```python
from build123d import *

# Parameters (mm, degrees)
SKETCH1_R           = 35
BOSS_EXTRUDE1_DEPTH = 150
FILLET1_R           = 1
CUT_EXTRUDE1_START  = -10
SKETCH3_R           = 35
SKETCH3_R_2         = 34
CUT_EXTRUDE1_DEPTH  = 10
BOSS_EXTRUDE2_START = -5
SKETCH4_R           = 2.25
BOSS_EXTRUDE2_DEPTH = 6
BOSS_EXTRUDE3_DEPTH = 64


with BuildPart() as part:
    # Sketch1 → Boss-Extrude1 (new body)
    with BuildSketch(Plane(origin=(0, 0, 0), x_dir=(1, 0, 0), z_dir=(0, 1, 0))):
        with Locations(Location((0, 0, 0), (0, 0, 270))):
            Circle(SKETCH1_R)
        with BuildLine():
            Line((-31.448370387, -10), (31.448370387, -10))
            ThreePointArc((31.448370387, -10), (0, 33), (-31.448370387, -10))
        make_face(mode=Mode.SUBTRACT)
        with BuildLine():
            Line((-30.740852298, -12), (30.740852298, -12))
            ThreePointArc((30.740852298, -12), (0, -33), (-30.740852298, -12))
        make_face(mode=Mode.SUBTRACT)
    extrude(amount=BOSS_EXTRUDE1_DEPTH)

    # Fillet1
    fillet1_edges = [part.edges().sort_by_distance(p)[0] for p in [
        (-30.740852298, 75, 12),
        (30.740852298, 75, 12),
        (31.448370387, 75, 10),
        (-31.448370387, 75, 10),
    ]]
    fillet(fillet1_edges, radius=FILLET1_R)

    # Sketch3 → Cut-Extrude1 (cut)
    # profile 1 of 2: a face of its own
    with BuildSketch(Plane(origin=(0, 150, 0), x_dir=(1, 0, 0), z_dir=(0, 1, 0)).offset(CUT_EXTRUDE1_START)):
        with Locations(Location((0, 0, 0), (0, 0, 270))):
            Circle(SKETCH3_R)
        with Locations(Location((0, 0, 0), (0, 0, 270))):
            Circle(SKETCH3_R_2, mode=Mode.SUBTRACT)
    # profile 2 of 2: a face of its own
    with BuildSketch(Plane(origin=(0, 150, 0), x_dir=(1, 0, 0), z_dir=(0, 1, 0)).offset(CUT_EXTRUDE1_START)):
        with BuildLine():
            Line((30.708305066, -10), (-30.708305066, -10))
            ThreePointArc((-30.708305066, -10), (-31.307784006, -9.80039053), (-31.667939599, -9.28125))
            ThreePointArc((-31.667939599, -9.28125), (-31.402080367, -10.144424508), (-31.112698372, -11))
            Line((-31.112698372, -11), (31.112698372, -11))
            ThreePointArc((31.112698372, -11), (31.402080367, -10.144424508), (31.667939599, -9.28125))
            ThreePointArc((31.667939599, -9.28125), (31.307784006, -9.80039053), (30.708305066, -10))
        make_face()
    extrude(amount=CUT_EXTRUDE1_DEPTH, mode=Mode.SUBTRACT)

    # Sketch4 → Boss-Extrude2 (add)
    with BuildSketch(Plane.XZ.offset(BOSS_EXTRUDE2_START)):
        with BuildLine():
            Line((-23.25, 10), (23.25, 10))
            Line((23.25, 10), (23.25, 0))
            ThreePointArc((23.25, 0), (19.66205807, -8.66205807), (11, -12.25))
            Line((11, -12.25), (7.5, -10.75))
            Line((7.5, -10.75), (-7.5, -10.75))
            Line((-7.5, -10.75), (-11, -12.25))
            ThreePointArc((-11, -12.25), (-19.66205807, -8.66205807), (-23.25, 0))
            Line((-23.25, 0), (-23.25, 10))
        make_face()
        with Locations(Location((0, -7.5, 0), (0, 0, 270))):
            Circle(SKETCH4_R, mode=Mode.SUBTRACT)
        with Locations(Location((20.5, 7.5, 0), (0, 0, 270))):
            Circle(SKETCH4_R, mode=Mode.SUBTRACT)
        with Locations(Location((-20.5, 7.5, 0), (0, 0, 270))):
            Circle(SKETCH4_R, mode=Mode.SUBTRACT)
        with Locations(Location((0, 7.5, 0), (0, 0, 270))):
            Circle(SKETCH4_R, mode=Mode.SUBTRACT)
        with BuildLine():
            Line((-3, 4.643543905), (3, 4.643543905))
            ThreePointArc((3, 4.643543905), (20.25, 0), (3, -4.643543905))
            Line((3, -4.643543905), (-3, -4.643543905))
            ThreePointArc((-3, -4.643543905), (-20.25, 0), (-3, 4.643543905))
        make_face(mode=Mode.SUBTRACT)
    extrude(amount=-BOSS_EXTRUDE2_DEPTH)

    # Sketch5 → Boss-Extrude3 (add)
    with BuildSketch(Plane(origin=(0, 11, 0), x_dir=(1, 0, 0), z_dir=(0, 1, 0))):
        with BuildLine():
            Line((-23.25, 0), (-23.25, -10))
            Line((-23.25, -10), (23.25, -10))
            Line((23.25, -10), (23.25, 0))
            ThreePointArc((23.25, 0), (19.66205807, 8.66205807), (11, 12.25))
            Line((11, 12.25), (7.5, 10.75))
            Line((7.5, 10.75), (-7.5, 10.75))
            Line((-7.5, 10.75), (-11, 12.25))
            ThreePointArc((-11, 12.25), (-19.66205807, 8.66205807), (-23.25, 0))
        make_face()
        with BuildLine():
            Line((3, -4.643543905), (-3, -4.643543905))
            ThreePointArc((-3, -4.643543905), (-20.25, 0), (-3, 4.643543905))
            Line((-3, 4.643543905), (3, 4.643543905))
            ThreePointArc((3, 4.643543905), (20.25, 0), (3, -4.643543905))
        make_face(mode=Mode.SUBTRACT)
    extrude(amount=BOSS_EXTRUDE3_DEPTH)


solid = part.part
```
Source: CAD feature listing. Evaluate the final solid. Frame: model axes, mm. A direction names the side the tool comes from. Coordinates: 2 decimals unless noted, no trailing zeros. Loops run counter-clockwise (first coordinate to the right, second up) from the corner with the lowest first, then second, coordinate; pieces in that order, holes last. Notation, with made-up numbers: (-31.5, -3.75) - (-13.5, -3.75) arc R29 cw to (-13.5, 21.25) - close; hole circle Ø2 at (4, -38). An arc over 180 degrees is marked (long way). Answer as CSV lines item,"result".
1. Section D-D (y = 15). Return loops of the section in (x, z), then the cut area to 3 significant figures.
Established:
outline,"circle Ø70 at (0, 0); hole (-31.67, 9.28) arc R33 ccw (long way) to (31.67, 9.28) arc R1 ccw to (30.71, 10) - (23.25, 10) - (23.25, 0) arc R12.25 cw to (11, -12.25) - (7.5, -10.75) - (-7.5, -10.75) - (-11, -12.25) arc R12.25 cw to (-23.25, 0) - (-23.25, 10) - (-30.71, 10) arc R1 ccw to start; hole (-30.15, 13.41) arc R1 ccw to (-29.24, 12) - (29.24, 12) arc R1 ccw to (30.15, 13.41) arc R33 ccw to start; hole (-3, -4.64) - (3, -4.64) arc R9.25 ccw (long way) to (3, 4.64) - (-3, 4.64) arc R9.25 ccw (long way) to start"
area,"918 mm2"
2. Mould query, pull axis X, two halves, no side actions, for faces 1 (the flat face through (0.2, 0, 10.2)), 2 (the flat face through (0, 11, -8)). Classes: released by +X, released by -X, zero draft, split by the parting line, or undercut.
Established:
face 1,"zero draft"
face 2,"undercut"
3. Contact query for flat-ended pins moving along their axis: pin 1 (8 mm diameter, centred on y = 37, z = 6, fed in from +X); pin 2 (1.5 mm diameter, centred on x = 14, y = 20.5, fed in from +Z) (3 decimals); pin 3 (3.5 mm diameter, centred on x = 0, z = -6.5, fed in from -Y); pin 4 (2 mm diameter, centred on x = -17.5, z = -24.5, fed in from -Y). Output: stop coordinate, or through.
Established:
pin 1,"stops at x = 34.94"
pin 2,"stops at z = 32.395"
pin 3,"stops at y = 5"
pin 4,"passes through"
4. Reachability of faces 3 (the cylindrical face through (-1.369, 7.958, 9.286)), 4 (the flat face through (-9.23, 39.51, -11.49)), 5 (the flat face through (0, 75, -6)) from +Z, -Z, +X, -X, +Y, -Y: full face, straight path, thin tool, end or side. Return the list, or none.
Established:
face 3,"-Y"
face 4,"+Y, -Y"
face 5,"+Y"
5. Section A-A (x = 0). Count the separate pieces of the cut face and the enclosed holes in it, then the cut area to 3 significant figures.
Established:
separate pieces,"4"
enclosed holes,"0"
area,"1,620 mm2"
6. Section C-C (x = -26). Return loops of the section in (y, z), then the cut area to 3 significant figures.
Established:
outline,"(0, -23.43) - (140, -23.43) - (140, -21.91) - (150, -21.91) - (150, -20.32) - (0, -20.32) - close; (0, 10) - (140, 10) - (140, 11) - (150, 11) - (150, 12) - (0, 12) - close; (0, 20.32) - (150, 20.32) - (150, 21.91) - (140, 21.91) - (140, 23.43) - (0, 23.43) - close"
area,"1,190 mm2"
7. Section B-B (y = 111.5). Return loops of the section in (x, z), then the cut area to 3 significant figures.
Established:
outline,"circle Ø70 at (0, 0); hole (-31.67, 9.28) arc R33 ccw (long way) to (31.67, 9.28) arc R1 ccw to (30.71, 10) - (-30.71, 10) arc R1 ccw to start; hole (-30.15, 13.41) arc R1 ccw to (-29.24, 12) - (29.24, 12) arc R1 ccw to (30.15, 13.41) arc R33 ccw to start"
area,"553 mm2"
8. Ray query, line 1 (Z direction, x = -3.5, y = 24.5); line 2 (X direction, y = 38.5, z = -4); line 3 (X direction, y = 39.5, z = -1). Return the intervals inside material, ascending.
Established:
line 1,"z = -34.82 to -32.81, -10.75 to -5.41, 5.41 to 12, 32.81 to 34.82"
line 2,"x = -34.77 to -32.76, -22.58 to -19.34, 19.34 to 22.58, 32.76 to 34.77"
line 3,"x = -34.99 to -32.98, -23.21 to -20.2, 20.2 to 23.21, 32.98 to 34.99"
